Model file for the job. Use its own axes, mm. A direction names the side the tool comes from. Give positions to 0.01 mm unless a question says otherwise; leave off trailing zeros. Loops run counter-clockwise (first coordinate to the right, second up) from the corner with the lowest first, then second, coordinate; pieces in that order, holes last. Notation, with made-up numbers: (-6, 78) - (41, 78) arc R35 ccw to (41, 110) - close; hole circle Ø3 at (36.25, -21). An arc over 180 degrees is marked (long way). Answer as CSV lines item,"result". Start each with the question number.
Item 1: Drill centre lines: L1, parallel to X at y = 6, z = 0; L2, parallel to X at y = 1.4, z = -22; L3, parallel to X at y = 5.5, z = 14.5. Where is each one in solid material? Low to high. Write a range as from..to.
Item 2: Pin check, flat tips, straight feed: pin 1 (6 mm diameter, centred on y = 13, z = 2, fed in from -X); pin 2 (1.5 mm diameter, centred on x = 11, z = -36.5, fed in from +Y); pin 3 (5 mm diameter, centred on x = -18.5, y = 9.5, fed in from -Z); pin 4 (3.5 mm diameter, centred on x = -36, z = -22, fed in from +Y). Stop position of each tip, or through.
Item 3: Saw through at A-A on x = 36. State how many separate pieces and enclosed holes the cut face has, plus the area to 3 significant figures.
Item 4: Tool access for faces 1 (the cylindrical face through (-43.028, 9.605, 22.38)), 2 (the cylindrical face through (34, 1, -22)), 3 (the cylindrical face through (50.85, 10.52, 1.67)): list every direction of +Z, -Z, +X, -X, +Y, -Y with a clear straight run to the whole face (end or side of a thin tool).
Item 5: Saw through at B-B on z = 22. Give the cut face in (x, y), plus the area to 3 significant figures.
Item 6: Saw through at D-D on x = -19.5. Give the cut face in (y, z).
Item 7: Pull direction X, two halves, no side cores. Call faces 4 (the cylindrical face through (-38, 1, -22)), 5 (the flat face through (-49.1, 13, 12.5)), 6 (the cylindrical face through (48.794, 6.409, -25.379)): pulls with the +X half, pulls with the -X half, needs draft (parallel to the pull), parting line crosses it, or undercut.
from build123d import *

# Parameters (mm, degrees)
SKETCH2_R                = 55
BOSS_EXTRUDE2_DEPTH      = 13
SKETCH7_R                = 50.5
BOSS_EXTRUDE3_DEPTH      = 4
SKETCH8_R                = 48.5
CUT_EXTRUDE3_DEPTH       = 15
SKETCH9_R                = 2
SKETCH9_W                = 3.162660916
SKETCH9_H                = 2.60493009
CUT_EXTRUDE4_DEPTH       = 15
CUT_EXTRUDE5_DEPTH       = 20
CUT_EXTRUDE5_DEPTH_BACK  = 1
SKETCH10_R               = 2.5
BOSS_EXTRUDE5_DEPTH      = 0.01
BOSS_EXTRUDE5_DEPTH_BACK = 2
SKETCH11_W               = 6.274273212
SKETCH11_H               = 7.379534018


with BuildPart() as part:
    # Sketch2 → Boss-Extrude2 (new body)
    with BuildSketch(Plane(origin=(0, 0, 0), x_dir=(1, 0, 0), z_dir=(0, 1, 0))):
        with Locations(Location((0, 0, 0), (0, 0, 90))):
            Circle(SKETCH2_R)
    extrude(amount=BOSS_EXTRUDE2_DEPTH)

    # Sketch7 → Boss-Extrude3 (add)
    with BuildSketch(Plane(origin=(0, 13, 0), x_dir=(1, 0, 0), z_dir=(0, 1, 0))):
        with Locations(Location((0, 0, 0), (0, 0, 270))):
            Circle(SKETCH7_R)
    extrude(amount=BOSS_EXTRUDE3_DEPTH)

    # Sketch8 → Cut-Extrude3 (cut)
    with BuildSketch(Plane(origin=(0, 17, 0), x_dir=(1, 0, 0), z_dir=(0, 1, 0))):
        with Locations(Location((0, 0, 0), (0, 0, 270))):
            Circle(SKETCH8_R)
    extrude(amount=-CUT_EXTRUDE3_DEPTH, mode=Mode.SUBTRACT)

    # Sketch9 → Cut-Extrude4 (cut)
    with BuildSketch(Plane(origin=(0, 2, 0), x_dir=(1, 0, 0), z_dir=(0, 1, 0))):
        with Locations(Location((36, -22, 0), (0, 0, 270))):
            Circle(SKETCH9_R)
        with Locations(Location((-36, 22, 0), (0, 0, 270))):
            Circle(SKETCH9_R)
        with Locations(Location((-35.8, -22, 0), (0, 0, 270))):
            Circle(SKETCH9_R)
        with Locations(Location((36, 22, 0), (0, 0, 270))):
            Circle(SKETCH9_R)
        with Locations((37.581330458, -0.802465045)):
            Rectangle(SKETCH9_W, SKETCH9_H)
    extrude(amount=-CUT_EXTRUDE4_DEPTH, mode=Mode.SUBTRACT)

    # Sketch10 → Cut-Extrude5 (cut, two sides: drawn at the far end of the back side and taken through both)
    with BuildSketch(Plane(origin=(36, 0, 0), x_dir=(0, 0, -1), z_dir=(1, 0, 0)).offset(-CUT_EXTRUDE5_DEPTH_BACK)):
        with Locations(Location((-2, 13, 0), (0, 0, 180))):
            Circle(SKETCH10_R)
    extrude(amount=CUT_EXTRUDE5_DEPTH + CUT_EXTRUDE5_DEPTH_BACK, mode=Mode.SUBTRACT)

    # Sketch11 → Boss-Extrude5 (add, two sides: drawn at the far end of the back side and taken through both)
    with BuildSketch(Plane(origin=(0, 2, 0), x_dir=(1, 0, 0), z_dir=(0, 1, 0)).offset(-BOSS_EXTRUDE5_DEPTH_BACK)):
        with Locations((37.193701051, -0.388212482)):
            Rectangle(SKETCH11_W, SKETCH11_H)
    extrude(amount=BOSS_EXTRUDE5_DEPTH + BOSS_EXTRUDE5_DEPTH_BACK)


solid = part.part
Responses:
1,L1,"-55..-48.5, 48.5..55"
1,L2,"-50.41..-38, -34..34, 38..50.41"
1,L3,"-53.05..-46.28, 46.28..53.05"
2,pin 1,"x = -55"
2,pin 2,"y = 2"
2,pin 3,"z = -52.62"
2,pin 4,"through"
3,separate pieces,"3"
3,enclosed holes,"0"
3,area,"374 mm2"
4,face 1,"+Y"
4,face 2,"+Y, -Y"
4,face 3,"+X"
5,outline,"(-50.41, 0) - (-37.8, 0) - (-37.8, 2) - (-43.22, 2) - (-43.22, 17) - (-45.46, 17) - (-45.46, 13) - (-50.41, 13) - close; (-33.8, 0) - (34, 0) - (34, 2) - (-33.8, 2) - close; (38, 0) - (50.41, 0) - (50.41, 13) - (45.46, 13) - (45.46, 17) - (43.22, 17) - (43.22, 2) - (38, 2) - close"
5,area,"362 mm2"
6,outline,"(0, -51.43) - (13, -51.43) - (13, -46.58) - (17, -46.58) - (17, -44.41) - (2, -44.41) - (2, 44.41) - (17, 44.41) - (17, 46.58) - (13, 46.58) - (13, 51.43) - (0, 51.43) - close"
7,face 4,"undercut"
7,face 5,"needs draft"
7,face 6,"parting line crosses it"
